For this review, take the finished solid that the model builds, in its own axes (mm). Face numbers are marked on the shaded views. Give positions to 0.01 mm unless a question says otherwise; leave off trailing zeros. Order: outer loops, then holes, each group sorted by start corner. A loop starts at its lowest first (then second) coordinate and runs counter-clockwise, first axis right, second up. Notation, with made-up numbers: (65.5, 54.25) - (87.5, 54.25) arc R23 cw to (87.5, 77.25) - close; hole circle Ø7 at (67.5, 11.5). An arc over 180 degrees is marked (long way). Answer as a JSON object with one key per item and string values. Group by question number.
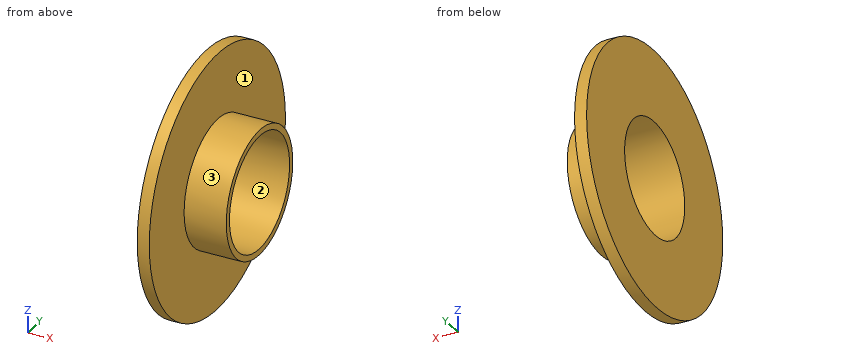
Autodesk Inventor part; units mm, degrees
ref_plane "YZ Plane" through (0, 0, 0) normal (1, 0, 0) x (0, 1, 0)
ref_plane "XZ Plane" through (0, 0, 0) normal (0, 1, 0) x (-1, 0, 0)
ref_plane "XY Plane" through (0, 0, 0) normal (0, 0, 1) x (1, 0, 0)
sketch "Sketch2" plane through (0, 0, 0) normal (1, 0, 0) x (0, 1, 0)
  circle A0 centre (0, 0) radius 21.5
  dimension "d3" = 43
extrude "Extrusion1" add sketch "Sketch2" along normal blind 2
sketch "Sketch3" plane through (2, 0, 0) normal (1, 0, 0) x (0, 0, -1)
  circle A0 centre (0, 0) radius 21.5
  circle A1 centre (0, 0) radius 9.5
  dimension "d6" = 19
extrude "Extrusion2" cut sketch "Sketch3" against normal blind 2 contours A1
sketch "Sketch4" plane through (2, 0, 0) normal (1, 0, 0) x (0, 0, -1)
  circle A0 centre (0, 0) radius 9.5
  circle A1 centre (0, 0) radius 21.5
  circle A2 centre (0, 0) radius 10.5
  dimension "d9" = 21
extrude "Extrusion3" add sketch "Sketch4" along normal blind 7 contours A2
properties part number "holeCover"
1) Mouldability with a two-part tool opening along Y and no side actions: class the marked faces 1, 2 and 3 as released by +Y, released by -Y, zero draft, split by the parting line, or undercut.
2) For pin 1 (1.5 mm diameter, centred on y = 15, z = -7.5, fed in from +X); pin 2 (3 mm diameter, centred on x = 1.5, y = 9.5, fed in from -Z); pin 3 (17 mm diameter, centred on y = 0, z = 0, fed in from +X), all flat-tipped, find the tip position at first contact; note any pin that passes through.
3) For line 1 (Y direction, x = 3, z = 0); line 2 (X direction, y = 3, z = -15.5); line 3 (Y direction, x = 7, z = -4), list the stretches that pass through material, from the lowest coordinate up.
4) Consider section C-C (x = 8.25). Give the boundary of the cut face in (y, z), plus the area to 3 significant figures.
5) Consider section A-A (z = 0). Give the boundary of the cut face in (x, y).
6) Consider section D-D (z = -17.5). Give the boundary of the cut face in (x, y).
Result set:
{
 "1": {"face 1": "zero draft", "face 2": "undercut", "face 3": "split by the parting line"},
 "2": {"pin 1": "stops at x = 2", "pin 2": "stops at z = -19.96", "pin 3": "passes through"},
 "3": {"line 1": "y = -10.5 to -9.5, 9.5 to 10.5", "line 2": "x = 0 to 2", "line 3": "y = -9.71 to -8.62, 8.62 to 9.71"},
 "4": {"outline": "circle Ø21 at (0, 0); hole circle Ø19 at (0, 0)", "area": "62.8 mm2"},
 "5": {"outline": "(0, -21.5) - (2, -21.5) - (2, -10.5) - (9, -10.5) - (9, -9.5) - (0, -9.5) - close; (0, 9.5) - (9, 9.5) - (9, 10.5) - (2, 10.5) - (2, 21.5) - (0, 21.5) - close"},
 "6": {"outline": "(0, -12.49) - (2, -12.49) - (2, 12.49) - (0, 12.49) - close"}
}
